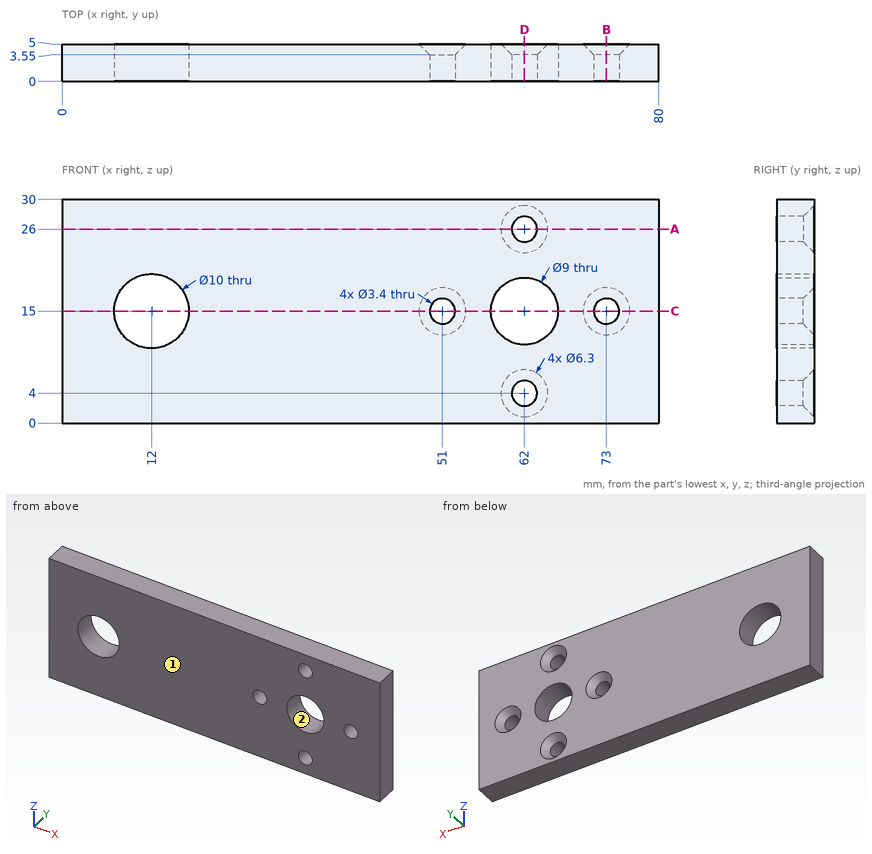
Geometry: see drawing. Coordinates: mm, zero at the bounding-box minimum. Round coordinates to 2 decimals unless told otherwise and drop trailing zeros. Write each loop counter-clockwise with the first axis right and the second up, starting at its lowest first coordinate (ties: lowest second). Pieces come first, ordered by that corner, then holes. Notation, with made-up numbers: M 42,-13 L 49,-13 A21 ccw 49,8 Z; hole C -16,-3.75 d8. An arc over 180 degrees is marked long. Answer in a Markdown table with one row per item. Add a question column.
(1) Cut plane D-D, the plane x = 62. Return the cut outline in (y, z), then the cut area to 3 significant figures.
(2) Cut plane B-B, the plane x = 73. Return the cut outline in (y, z).
(3) Cut plane A-A, the plane z = 26. Return the cut outline in (x, y), then the cut area to 3 significant figures.
(4) Contact query for a flat-ended pin moving along its axis: pin 1 (7 mm diameter, centred on x = 62, z = 15, fed in from -Y). Output: stop coordinate, or through.
(5) Ray query, L1, parallel to X at y = 2.95, z = 13.25; L2, parallel to X at y = 1.2, z = 4; L3, parallel to Z at x = 73, y = 1.15. Return the intervals inside material, ascending.
(6) Draft query along Z for the marked faces 1 and 2. Return one class per face: pulls with the +Z half, pulls with the -Z half, needs draft (parallel to the pull), parting line crosses it, or undercut.
(7) Cut plane C-C, the plane z = 15. Return the cut outline in (x, y), then the cut area to 3 significant figures.
Established:
| question | item | result |
|---|---|---|
| 1 | outline | M 0,0 L 5,0 L 5,0.85 L 3.55,2.3 L 0,2.3 Z; M 0,5.7 L 3.55,5.7 L 5,7.15 L 5,10.5 L 0,10.5 Z; M 0,19.5 L 5,19.5 L 5,22.85 L 3.55,24.3 L 0,24.3 Z; M 0,27.7 L 3.55,27.7 L 5,29.15 L 5,30 L 0,30 Z |
| 1 | area | 66.8 mm² |
| 2 | outline | M 0,0 L 5,0 L 5,11.85 L 3.55,13.3 L 0,13.3 Z; M 0,16.7 L 3.55,16.7 L 5,18.15 L 5,30 L 0,30 Z |
| 3 | outline | M 0,0 L 60.3,0 L 60.3,3.55 L 58.85,5 L 0,5 Z; M 63.7,0 L 80,0 L 80,5 L 65.15,5 L 63.7,3.55 Z |
| 3 | area | 381 mm² |
| 4 | pin 1 | through |
| 5 | L1 | 0 to 7.32, 16.68 to 57.85, 66.15 to 80 |
| 5 | L2 | 0 to 60.3, 63.7 to 80 |
| 5 | L3 | 0 to 13.3, 16.7 to 30 |
| 6 | face 1 | needs draft |
| 6 | face 2 | undercut |
| 7 | outline | M 0,0 L 7,0 L 7,5 L 0,5 Z; M 17,0 L 49.3,0 L 49.3,3.55 L 47.85,5 L 17,5 Z; M 52.7,0 L 57.5,0 L 57.5,5 L 54.15,5 L 52.7,3.55 Z; M 66.5,0 L 71.3,0 L 71.3,3.55 L 69.85,5 L 66.5,5 Z; M 74.7,0 L 80,0 L 80,5 L 76.15,5 L 74.7,3.55 Z |
| 7 | area | 267 mm² |
